Could you check a few things on this model? Use its own coordinates, in mm. Round coordinates to 2 decimals unless told otherwise and drop trailing zeros. Loops run counter-clockwise (first coordinate to the right, second up) from the corner with the lowest first, then second, coordinate; pieces in that order, holes last. Notation, with made-up numbers: (60.5, 18) -> (77.5, 18) arc R19 ccw to (77.5, 43) -> close; hole circle Ø10 at (10.25, 69.5). An arc over 180 degrees is marked (long way). One line per item, written item: value.
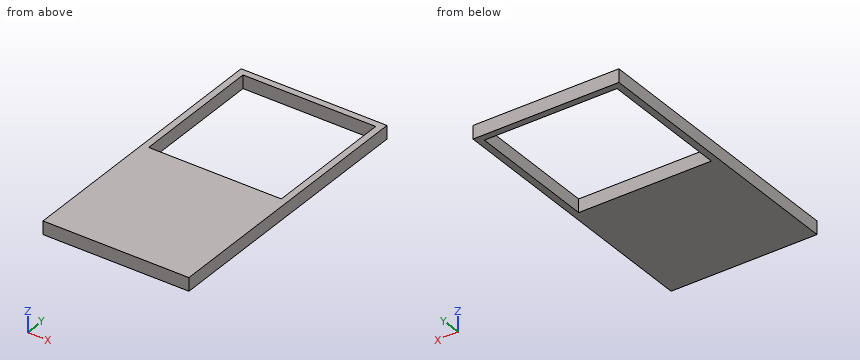
from build123d import *

# Parameters (mm, degrees)
SKETCH1_W           = 27.94
SKETCH1_H           = 27.94
SKETCH1_W_2         = 25.4
SKETCH1_H_2         = 25.4
EXTRUDE_THIN1_DEPTH = 1.27
SKETCH2_W           = 27.94
SKETCH2_H           = 25.4
BOSS_EXTRUDE1_DEPTH = 2.54


with BuildPart() as part:
    # Sketch1 → Extrude-Thin1 (new body, symmetric)
    with BuildSketch(Plane.XY):
        Rectangle(SKETCH1_W, SKETCH1_H)
        Rectangle(SKETCH1_W_2, SKETCH1_H_2, mode=Mode.SUBTRACT)
    extrude(amount=EXTRUDE_THIN1_DEPTH, both=True)

    # Sketch2 → Boss-Extrude1 (add, through all)
    with BuildSketch(Plane.XY.offset(1.27)):
        with Locations((0, -26.67)):
            Rectangle(SKETCH2_W, SKETCH2_H)
    extrude(amount=-BOSS_EXTRUDE1_DEPTH)


solid = part.part
(1) If we section it at C-C, the plane z = 0.3: Please give me the cut outline in (x, y), then the cut area to 3 significant figures.
Recorded:
outline: (-13.97, -39.37) -> (13.97, -39.37) -> (13.97, 13.97) -> (-13.97, 13.97) -> close; hole (-12.7, -12.7) -> (12.7, -12.7) -> (12.7, 12.7) -> (-12.7, 12.7) -> close
area: 845 mm²
(2) If we section it at B-B, the plane x = -5.75: Please give me the cut outline in (y, z), then the cut area to 3 significant figures.
Recorded:
outline: (-39.37, -1.27) -> (-12.7, -1.27) -> (-12.7, 1.27) -> (-39.37, 1.27) -> close; (12.7, -1.27) -> (13.97, -1.27) -> (13.97, 1.27) -> (12.7, 1.27) -> close
area: 71.0 mm²
(3) If we section it at A-A, the plane y = 3.5: Please give me the cut outline in (x, z), then the cut area to 3 significant figures.
Recorded:
outline: (-13.97, -1.27) -> (-12.7, -1.27) -> (-12.7, 1.27) -> (-13.97, 1.27) -> close; (12.7, -1.27) -> (13.97, -1.27) -> (13.97, 1.27) -> (12.7, 1.27) -> close
area: 6.45 mm²
(4) If I drill on L1, parallel to Y at x = 9, z = 1.05; L2, parallel to X at y = 12, z = -0.7, over which ranges is the centre line in solid material (lowest first)?
Recorded:
L1: -39.37 to -12.7, 12.7 to 13.97
L2: -13.97 to -12.7, 12.7 to 13.97
